```python
from build123d import *

# Parameters (mm, degrees)
BOSS_EXTRUDE1_DEPTH = 88.9
CUT_EXTRUDE1_DEPTH  = 203.2
BOSS_EXTRUDE2_DEPTH = 31.75
SKETCH5_R           = 7.9375
CUT_EXTRUDE2_DEPTH  = 31.75
SKETCH6_R           = 4.7625
BOSS_EXTRUDE3_DEPTH = 9.525


with BuildPart() as part:
    # Sketch2 → Boss-Extrude1 (new body)
    with BuildSketch(Plane(origin=(0, 0, 0), x_dir=(0, 0, -1), z_dir=(1, 0, 0))):
        with BuildLine():
            Line((0, 0), (0, 66.675))
            ThreePointArc((0, 66.675), (6.227207921, 87.549269451), (22.873234913, 101.6))
            Line((22.873234913, 101.6), (38.1, 101.6))
            Line((38.1, 101.6), (38.1, 50.8))
            Line((38.1, 50.8), (171.45, 50.8))
            Line((171.45, 50.8), (171.45, 76.2))
            Line((171.45, 76.2), (203.2, 76.2))
            Line((203.2, 76.2), (203.2, 0))
            Line((203.2, 0), (171.45, 0))
            Line((171.45, 0), (38.1, 0))
            Line((38.1, 0), (0, 0))
        make_face()
    extrude(amount=BOSS_EXTRUDE1_DEPTH)

    # Sketch3 → Cut-Extrude1 (cut)
    with BuildSketch(Plane(origin=(0, 0, -203.2), x_dir=(-1, 0, 0), z_dir=(0, 0, -1))):
        Polygon((-44.45, 0), (-25.4, 0), (-25.4, 31.75), (-28.575, 31.75), (-28.575, 53.975), (-60.325, 53.975), (-60.325, 31.75), (-63.5, 31.75), (-63.5, 0), align=None)
    extrude(amount=-CUT_EXTRUDE1_DEPTH, mode=Mode.SUBTRACT)

    # Sketch4 → Boss-Extrude2 (add)
    with BuildSketch(Plane(origin=(0, 0, -203.2), x_dir=(-1, 0, 0), z_dir=(0, 0, -1))):
        with BuildLine():
            Line((-63.5, 76.2), (-25.4, 76.2))
            ThreePointArc((-25.4, 76.2), (-44.45, 95.25), (-63.5, 76.2))
        make_face()
    extrude(amount=-BOSS_EXTRUDE2_DEPTH)

    # Sketch5 → Cut-Extrude2 (cut)
    with BuildSketch(Plane(origin=(0, 0, -203.2), x_dir=(-1, 0, 0), z_dir=(0, 0, -1))):
        with Locations((-44.45, 76.2)):
            Circle(SKETCH5_R)
    extrude(amount=-CUT_EXTRUDE2_DEPTH, mode=Mode.SUBTRACT)

    # Sketch6 → Boss-Extrude3 (add)
    with BuildSketch(Plane(origin=(0, 0, 0), x_dir=(1, 0, 0), z_dir=(0, 1, 0))):
        with BuildLine():
            ThreePointArc((-22.831460674, 23.830337079), (-31.75, 38.1), (-22.831460674, 52.369662921))
            Line((-22.831460674, 52.369662921), (0, 63.5))
            Line((0, 63.5), (0, 12.7))
            Line((0, 12.7), (-22.831460674, 23.830337079))
        make_face()
        with Locations((-15.875, 38.1)):
            Circle(SKETCH6_R, mode=Mode.SUBTRACT)
        with BuildLine():
            ThreePointArc((-22.831460674, 150.830337079), (-31.75, 165.1), (-22.831460674, 179.369662921))
            Line((-22.831460674, 179.369662921), (0, 190.5))
            Line((0, 190.5), (0, 139.7))
            Line((0, 139.7), (-22.831460674, 150.830337079))
        make_face()
        with Locations((-15.875, 165.1)):
            Circle(SKETCH6_R, mode=Mode.SUBTRACT)
        with BuildLine():
            Line((88.9, 139.7), (111.731460674, 150.830337079))
            ThreePointArc((111.731460674, 150.830337079), (120.65, 165.1), (111.731460674, 179.369662921))
            Line((111.731460674, 179.369662921), (88.9, 190.5))
            Line((88.9, 190.5), (88.9, 139.7))
        make_face()
        with Locations((104.775, 165.1)):
            Circle(SKETCH6_R, mode=Mode.SUBTRACT)
        with BuildLine():
            Line((88.9, 12.7), (111.731460674, 23.830337079))
            ThreePointArc((111.731460674, 23.830337079), (120.65, 38.1), (111.731460674, 52.369662921))
            Line((111.731460674, 52.369662921), (88.9, 63.5))
            Line((88.9, 63.5), (88.9, 12.7))
        make_face()
        with Locations((104.775, 38.1)):
            Circle(SKETCH6_R, mode=Mode.SUBTRACT)
    extrude(amount=BOSS_EXTRUDE3_DEPTH)


solid = part.part
```
Read the model definition and answer for the solid it produces. Units are mm, in the model's axes. A direction names the side the tool comes from. Give positions to 0.01 mm unless a question says otherwise; leave off trailing zeros. Write each loop counter-clockwise with the first axis right and the second up, starting at its lowest first coordinate (ties: lowest second). Pieces come first, ordered by that corner, then holes. Notation, with made-up numbers: M 48,-12.5 L 58,-12.5 A15 cw 58,15.5 Z; hole C 35.5,16.5 d7. An arc over 180 degrees is marked long. Put each result on its own line as item: value. Start each with the question number.
1. Each of these flat-tipped pins is pushed along its axis until it touches: pin 1 Ø12.5 at (x, z) = (12, -185) entering from +Y; pin 2 Ø1.5 at (y, z) = (34, -74) entering from -X; pin 3 Ø11 at (x, z) = (-15.875, -165.1) entering from +Y (3 decimals); pin 4 Ø3 at (x, z) = (31, -59.5) entering from -Y (3 decimals). Where does it stop, or does it pass through?
2. Consider line 1 along X through (y, z) = (6.5, -165.1); line 2 along X through (y, z) = (5.5, -66.5); line 3 along X through (y, z) = (52.5, -10) (3 decimals). Determine where each line is inside the solid, lowest interval first.
3. For a pull along Y with two mould halves and no side action, classify faces 6 (the flat face through (74, 50.8, -104)), 7 (the cylindrical face through (50.3, 81.565, -187.547)), 8 (the flat face through (-11.26, 4.7, -18.19)) as released by +Y, released by -Y, zero draft, split by the parting line, or undercut.
4. The part is cut by section C-C, the plane z = -71.5. Give the vertices of the cut face in (x, y) (3 decimals).
5. The part is cut by section B-B, the plane y = 43. Give the vertices of the cut face in (x, z) (3 decimals).
6. The part is cut by section A-A, the plane z = -165.1. Give the number of separate pieces and of enclosed holes in the cut face, and give its area (4 significant figures).
7. Which of the six approach directions +Z, -Z, +X, -X, +Y, -Y give full straight-line access (tool end or side, diameter ignored) to faces 1 (the flat face through (-11.576, 4.696, -57.857)), 2 (the flat face through (97, 9.525, -38)), 3 (the flat face through (63.5, 16, -103)), 4 (the flat face through (76, 76.2, -187)), 5 (the flat face through (44, 77, -38.1))?
8. The part is cut by section D-D, the plane x = 75. Give the vertices of the cut face in (y, z) (3 decimals), and give its area (3 significant figures).
Final values:
1. pin 1: stops at y = 76.2
1. pin 2: stops at x = 0
1. pin 3: stops at y = 9.525
1. pin 4: passes through
2. line 1: x = -31.75 to -20.64, -11.11 to 25.4, 63.5 to 100.01, 109.54 to 120.65
2. line 2: x = 0 to 25.4, 63.5 to 88.9
2. line 3: x = 0 to 28.575, 60.325 to 88.9
3. face 6: released by +Y
3. face 7: undercut
3. face 8: zero draft
4. outline: M 0,0 L 25.4,0 L 25.4,31.75 L 28.575,31.75 L 28.575,50.8 L 0,50.8 Z; M 60.325,31.75 L 63.5,31.75 L 63.5,0 L 88.9,0 L 88.9,50.8 L 60.325,50.8 Z
5. outline: M 0,-203.2 L 28.575,-203.2 L 28.575,0 L 0,0 Z; M 60.325,-203.2 L 88.9,-203.2 L 88.9,0 L 60.325,0 Z
6. separate pieces: 4
6. enclosed holes: 0
6. area: 3,125 mm²
7. face 1: -X, +Y, -Y
7. face 2: +Z, -Z, +X, +Y
7. face 3: +Z, -Z, -Y
7. face 4: -Z, +X, +Y
7. face 5: +X, -X, +Y
8. outline: M 0,-203.2 L 76.2,-203.2 L 76.2,-171.45 L 50.8,-171.45 L 50.8,-38.1 L 101.6,-38.1 L 101.6,-22.873 A38.1 ccw 66.675,0 L 0,0 Z
8. area: 12,800 mm²
